from build123d import *

# Parameters (mm, degrees)
F1_DEPTH = 19.05


with BuildPart() as f1:
    # F0 (on Front) → F1 (new body)
    with BuildSketch(Plane.XZ):
        with BuildLine():
            Line((-160.187716, -40.682596), (-25.399898, -40.682596))
            ThreePointArc((-25.399898, -40.682596), (0, -15.282697), (25.399898, -40.682596))
            Line((25.399898, -40.682596), (160.187742, -40.682596))
            Line((160.187742, -40.682596), (160.187742, 40.682596))
            Line((160.187742, 40.682596), (-160.187716, 40.682596))
            Line((-160.187716, 40.682596), (-160.187716, -40.682596))
        make_face()
        with BuildLine():
            ThreePointArc((-109.387919, 3.767226), (-115.737894, 10.117201), (-109.387919, 16.467176))
            Line((-109.387919, 16.467176), (-83.988021, 16.467176))
            ThreePointArc((-83.988021, 16.467176), (-77.638046, 10.117201), (-83.988021, 3.767226))
            Line((-83.988021, 3.767226), (-109.387919, 3.767226))
        make_face(mode=Mode.SUBTRACT)
        with BuildLine():
            ThreePointArc((-12.699949, 3.767226), (-19.049924, 10.117201), (-12.699949, 16.467176))
            Line((-12.699949, 16.467176), (12.699949, 16.467176))
            ThreePointArc((12.699949, 16.467176), (19.049924, 10.117201), (12.699949, 3.767226))
            Line((12.699949, 3.767226), (-12.699949, 3.767226))
        make_face(mode=Mode.SUBTRACT)
        with BuildLine():
            ThreePointArc((109.387945, 16.467176), (115.737919, 10.117201), (109.387945, 3.767226))
            Line((109.387945, 3.767226), (83.988021, 3.767226))
            ThreePointArc((83.988021, 3.767226), (77.638046, 10.117201), (83.988021, 16.467176))
            Line((83.988021, 16.467176), (109.387945, 16.467176))
        make_face(mode=Mode.SUBTRACT)
    extrude(amount=F1_DEPTH)


solid = f1.part
Here's how the part is built. I have some questions about the finished solid (model axes, mm). A direction names the side the tool comes from. Coordinates: 2 decimals unless noted, no trailing zeros. Loops run counter-clockwise (first coordinate to the right, second up) from the corner with the lowest first, then second, coordinate; pieces in that order, holes last. Notation, with made-up numbers: (85.25, 7) -> (117.25, 7) arc R20 cw to (117.25, 40) -> close; hole circle Ø10 at (-35, 61.25). An arc over 180 degrees is marked (long way). Use one line per item in the form item = value. Start each with the question number.
(1) Will this pin go through, and if not, where does the flat tip stop? pin 1 (5.5 mm diameter, centred on x = -1.5, y = -7, fed in from -Z).
(2) If we section it at A-A (x = 91.5): Please give me the cut outline in (y, z).
(3) Please list where these lines run through material, in increasing order: line 1 along X through (y, z) = (-4, 10); line 2 along X through (y, z) = (-12, 8); line 3 along Z through (x, y) = (88, -7).
(4) We'd pull the mould along X, two halves only. Please class faces 1 (the face through (115.736, -9.392, 10.257)), 2 (the face through (2, -9, 40.683)), 3 (the face through (160.188, -9, -1)): pulls with the +X half, pulls with the -X half, needs draft (parallel to the pull), parting line crosses it, or undercut.
(5) If we section it at C-C (z = -22): Please give me the cut outline in (x, y).
(6) If we section it at B-B (y = -13.5): Please give me the cut outline in (x, z).
(7) On a 3-axis mill with a long thin cutter (end or side, diameter ignored), from which of +Z, -Z, +X, -X, +Y, -Y can I reach the whole of each face in a straight line? I mean faces 4 (the face through (97, -9, 3.767)), 5 (the face through (-0.56, -9.39, -15.29)). Say none if no direction works.
Verdict:
q1.pin_1 = -15.64
q2.outline = (-19.05, -40.68) -> (0, -40.68) -> (0, 3.77) -> (-19.05, 3.77) -> close; (-19.05, 16.47) -> (0, 16.47) -> (0, 40.68) -> (-19.05, 40.68) -> close
q3.line_1 = -160.19 to -115.74, -77.64 to -19.05, 19.05 to 77.64, 115.74 to 160.19
q3.line_2 = -160.19 to -115.37, -78 to -18.69, 18.69 to 78, 115.37 to 160.19
q3.line_3 = -40.68 to 3.77, 16.47 to 40.68
q4.face_1 = undercut
q4.face_2 = needs draft
q4.face_3 = pulls with the +X half
q5.outline = (-160.19, -19.05) -> (-17.21, -19.05) -> (-17.21, 0) -> (-160.19, 0) -> close; (17.21, -19.05) -> (160.19, -19.05) -> (160.19, 0) -> (17.21, 0) -> close
q6.outline = (-160.19, -40.68) -> (-25.4, -40.68) arc R25.4 cw to (25.4, -40.68) -> (160.19, -40.68) -> (160.19, 40.68) -> (-160.19, 40.68) -> close; hole (-109.39, 3.77) -> (-83.99, 3.77) arc R6.35 ccw to (-83.99, 16.47) -> (-109.39, 16.47) arc R6.35 ccw to start; hole (-12.7, 3.77) -> (12.7, 3.77) arc R6.35 ccw to (12.7, 16.47) -> (-12.7, 16.47) arc R6.35 ccw to start; hole (83.99, 3.77) -> (109.39, 3.77) arc R6.35 ccw to (109.39, 16.47) -> (83.99, 16.47) arc R6.35 ccw to start
q7.face_4 = +Y, -Y
q7.face_5 = -Z, +Y, -Y
